```python
from build123d import *

# Parameters (mm, degrees)
SKETCH1_R           = 25
BOSS_EXTRUDE1_DEPTH = 2.5
SCALE1_SCALE        = 1.5


with BuildPart() as part:
    # Sketch1 → Boss-Extrude1 (new, symmetric)
    with BuildSketch(Plane.XY):
        with BuildLine():
            Line((0, 32.5), (-2.980263218, 27.338032686))
            ThreePointArc((-2.980263218, 27.338032686), (-9.904736181, 25.654360276), (-16.164094438, 22.247967345))
            Line((-16.164094438, 22.247967345), (-16.75283521, 27.849461618))
            ThreePointArc((-16.75283521, 27.849461618), (-17.944809925, 27.096748823), (-19.1030207, 26.293052317))
            Line((-19.1030207, 26.293052317), (-18.479976031, 20.365178268))
            ThreePointArc((-18.479976031, 20.365178268), (-23.092354522, 14.932955588), (-26.154054198, 8.497967345))
            Line((-26.154054198, 8.497967345), (-29.922831212, 12.683618263))
            ThreePointArc((-29.922831212, 12.683618263), (-30.444725533, 11.374035661), (-30.90933678, 10.043052317))
            Line((-30.90933678, 10.043052317), (-26.920966111, 5.613517939))
            ThreePointArc((-26.920966111, 5.613517939), (-27.459478317, -1.492330582), (-26.154054198, -8.497967345))
            Line((-26.154054198, -8.497967345), (-31.663322731, -7.326936169))
            ThreePointArc((-31.663322731, -7.326936169), (-31.315790766, -8.693172534), (-30.90933678, -10.043052317))
            Line((-30.90933678, -10.043052317), (-25.079062147, -11.282315447))
            ThreePointArc((-25.079062147, -11.282315447), (-21.338014708, -17.347597192), (-16.164094438, -22.247967345))
            Line((-16.164094438, -22.247967345), (-21.309501164, -24.538850017))
            ThreePointArc((-21.309501164, -24.538850017), (-20.225288311, -25.439884291), (-19.1030207, -26.293052317))
            Line((-19.1030207, -26.293052317), (-13.657808848, -23.868687803))
            ThreePointArc((-13.657808848, -23.868687803), (-7.066154732, -26.576671298), (0, -27.5))
            Line((0, -27.5), (-2.816174435, -32.377757204))
            ThreePointArc((-2.816174435, -32.377757204), (-1.409413153, -32.469424919), (0, -32.5))
            Line((0, -32.5), (2.980263218, -27.338032686))
            ThreePointArc((2.980263218, -27.338032686), (9.904736181, -25.654360276), (16.164094438, -22.247967345))
            Line((16.164094438, -22.247967345), (16.75283521, -27.849461618))
            ThreePointArc((16.75283521, -27.849461618), (17.944809925, -27.096748823), (19.1030207, -26.293052317))
            Line((19.1030207, -26.293052317), (18.479976031, -20.365178268))
            ThreePointArc((18.479976031, -20.365178268), (23.092354522, -14.932955588), (26.154054198, -8.497967345))
            Line((26.154054198, -8.497967345), (29.922831212, -12.683618263))
            ThreePointArc((29.922831212, -12.683618263), (30.444725533, -11.374035661), (30.90933678, -10.043052317))
            Line((30.90933678, -10.043052317), (26.920966111, -5.613517939))
            ThreePointArc((26.920966111, -5.613517939), (27.459478317, 1.492330582), (26.154054198, 8.497967345))
            Line((26.154054198, 8.497967345), (31.663322731, 7.326936169))
            ThreePointArc((31.663322731, 7.326936169), (31.315790766, 8.693172534), (30.90933678, 10.043052317))
            Line((30.90933678, 10.043052317), (25.079062147, 11.282315447))
            ThreePointArc((25.079062147, 11.282315447), (21.338014708, 17.347597192), (16.164094438, 22.247967345))
            Line((16.164094438, 22.247967345), (21.309501164, 24.538850017))
            ThreePointArc((21.309501164, 24.538850017), (20.225288311, 25.439884291), (19.1030207, 26.293052317))
            Line((19.1030207, 26.293052317), (13.657808848, 23.868687803))
            ThreePointArc((13.657808848, 23.868687803), (7.066154732, 26.576671298), (0, 27.5))
            Line((0, 27.5), (2.816174435, 32.377757204))
            ThreePointArc((2.816174435, 32.377757204), (1.409413153, 32.469424919), (0, 32.5))
        make_face()
        Circle(SKETCH1_R, mode=Mode.SUBTRACT)
    extrude(amount=BOSS_EXTRUDE1_DEPTH, both=True)


with BuildPart() as part_1:
    # Scale1: scaled about (0, 0, 0)
    add(part.part.scale(SCALE1_SCALE))


solid = part_1.part
```
Work out the finished part from the listing and answer in its coordinate system (mm). A direction names the side the tool comes from. Round coordinates to 2 decimals unless told otherwise and drop trailing zeros. Write each loop counter-clockwise with the first axis right and the second up, starting at its lowest first coordinate (ties: lowest second). Pieces come first, ordered by that corner, then holes. Notation, with made-up numbers: (-10, 45.5) -> (23, 45.5) arc R6 cw to (23, 53.5) -> close; hole circle Ø9 at (80, 54). An arc over 180 degrees is marked (long way). Write each question's results on one line, items separated by ' | '.
Q1. Flat-ended cylindrical pins translate along their axes: P1, Ø12, axis at x = 5.5, y = -31.5, coming from the +Z side; P2, Ø4, axis at x = -35, z = -0.5, coming from the -Y side; P3, Ø1, axis at x = 33, z = 0, coming from the +Y side; P4, Ø3, axis at y = 32, z = -2, coming from the -X side. Find the tip coordinate at first contact, or state that the pin passes through.
Data:
P1: z = 3.75 | P2: y = -24.75 | P3: y = 25.4 | P4: x = -28.03
Q2. Section D-D, the plane x = -30.5 is taken. Write down the section's boundary in (y, z), then the cut area to 3 significant figures.
Data:
outline: (-38.03, -3.75) -> (-36.16, -3.75) -> (-36.16, 3.75) -> (-38.03, 3.75) -> close; (-27.77, -3.75) -> (-21.82, -3.75) -> (-21.82, 3.75) -> (-27.77, 3.75) -> close; (21.82, -3.75) -> (27.77, -3.75) -> (27.77, 3.75) -> (21.82, 3.75) -> close | area: 103 mm^2
Q3. Section A-A, the plane y = 0 is taken. Write down the section's boundary in (x, z), then the cut area to 4 significant figures.
Data:
outline: (-41.25, -3.75) -> (-37.5, -3.75) -> (-37.5, 3.75) -> (-41.25, 3.75) -> close; (37.5, -3.75) -> (41.25, -3.75) -> (41.25, 3.75) -> (37.5, 3.75) -> close | area: 56.25 mm^2
Q4. Straight lines are drawn through the part: line 1 along Y through (x, z) = (0.5, 2); line 2 along X through (y, z) = (-34, -3); line 3 along X through (y, z) = (-27, 2.5). For each, find the intervals that lie inside material, in ascending order. Write a range as [from, to].
Data:
line 1: [-47.88, -37.5], [37.5, 41.25], [42.12, 48.75] | line 2: [-25.66, -15.82], [15.82, 23.36], [24.31, 28.08] | line 3: [-31.19, -26.02], [26.02, 31.19]
Q5. Section C-C, the plane x = -19 is taken. Write down the section's boundary in (y, z).
Data:
outline: (-36.61, -3.75) -> (-32.33, -3.75) -> (-32.33, 3.75) -> (-36.61, 3.75) -> close; (32.33, -3.75) -> (36.61, -3.75) -> (36.61, 3.75) -> (32.33, 3.75) -> close
Q6. Section B-B, the plane x = 1.5 is taken. Write down the section's boundary in (y, z).
Data:
outline: (-46.15, -3.75) -> (-37.47, -3.75) -> (-37.47, 3.75) -> (-46.15, 3.75) -> close; (37.47, -3.75) -> (41.22, -3.75) -> (41.22, 3.75) -> (37.47, 3.75) -> close; (43.85, -3.75) -> (48.73, -3.75) -> (48.73, 3.75) -> (43.85, 3.75) -> close
Q7. Determine the mould class of faces 5 (the cylindrical face through (14.717, -38.535, 0.053)), 6 (the cylindrical face through (30.36, 38.14, 0.05)), 7 (the flat face through (24.68, -37.51, 0.05)), 8 (the flat face through (-28.2, 35.1, 0.1)) for opening direction X: released by +X, released by -X, zero draft, split by the parting line, or undercut.
Data:
face 5: undercut | face 6: released by +X | face 7: undercut | face 8: released by -X
Q8. Which of the six approach directions +Z, -Z, +X, -X, +Y, -Y give full straight-line access (tool end or side, diameter ignored) to faces 1 (the cylindrical face through (-45.657, 17.089, 0.053)), 2 (the flat face through (-28.051, -35.066, 0.053)), 3 (the flat face through (43.31, 11.88, 0.05)), 4 (the flat face through (-24.628, -37.647, 0.053))?
Data:
face 1: +Z, -Z, -X, +Y | face 2: +Z, -Z, -X | face 3: +Z, -Z | face 4: +Z, -Z, -Y
